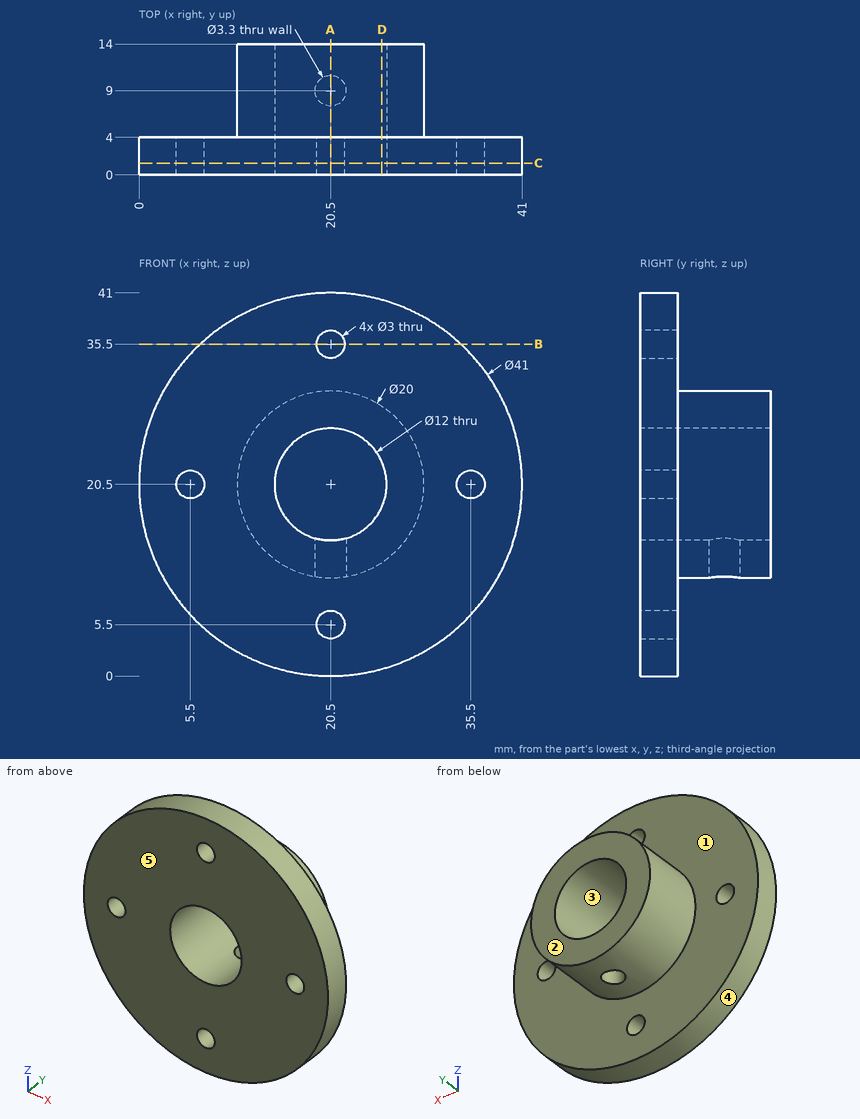
The drawing under review shows one solid part. Ordinate dimensions are in mm from its lowest x, y, z. A direction names the side the tool comes from. Coordinates: 2 decimals unless noted, no trailing zeros. Order: outer loops, then holes, each group sorted by start corner. A loop starts at its lowest first (then second) coordinate and runs counter-clockwise, first axis right, second up. Notation, with made-up numbers: M 56,-6.75 L 106,-6.75 A35 ccw 106,25.25 Z; hole C -30,57 d5. An arc over 180 degrees is marked long. Use a Markdown table: item, result.
(1) Add section B-B (z = 35.5). Give the boundary of the cut face in (x, y), then the cut area to 3 significant figures.
Worked answers:
| item | result |
|---|---|
| outline | M 6.53,0 L 19,0 L 19,4 L 6.53,4 Z; M 22,0 L 34.47,0 L 34.47,4 L 22,4 Z |
| area | 99.8 mm2 |
(2) Wall thickness on probe 1 along X at (y, z) = (3.15, 20.5); probe 2 along Z at (x, y) = (20.5, 7); probe 3 along Y at (x, z) = (20.5, 11.85): over which ranges is each line inside the solid? List them lowest first.
Worked answers:
| item | result |
|---|---|
| probe 1 | x = 0 to 4, 7 to 14.5, 26.5 to 34, 37 to 41 |
| probe 2 | z = 10.5 to 14.5, 26.5 to 30.5 |
| probe 3 | y = 0 to 7.35, 10.65 to 14 |
(3) For the marked faces 1 and 2, list the 3-axis set-ups (+Z, -Z, +X, -X, +Y, -Y) from which the entire face can be reached by the end or side of a thin tool; tool diameter is ignored.
Worked answers:
| item | result |
|---|---|
| face 1 | +Y |
| face 2 | +Z, -Z, +X, -X, +Y |
(4) Draft analysis for pull direction X (two halves, no side actions). For the marked faces 3, 4 and 5, state which applies: released by +X, released by -X, zero draft, split by the parting line, or undercut.
Worked answers:
| item | result |
|---|---|
| face 3 | undercut |
| face 4 | split by the parting line |
| face 5 | zero draft |
(5) Add section C-C (y = 1.25). Give the boundary of the cut face in (x, z).
Worked answers:
| item | result |
|---|---|
| outline | C 20.5,20.5 d41; hole C 5.5,20.5 d3; hole C 20.5,20.5 d12; hole C 20.5,5.5 d3; hole C 20.5,35.5 d3; hole C 35.5,20.5 d3 |
(6) For P1, Ø1, axis at y = 11, z = 11.5, coming from the -X side; P2, Ø1, axis at y = 5.5, z = 19, coming from the -X side; P3, Ø4, axis at x = 20.5, y = 9, coming from the +Z side, all flat-tipped, find the tip position at first contact; note any pin that passes through.
Worked answers:
| item | result |
|---|---|
| P1 | stops at x = 15.23 |
| P2 | stops at x = 10.55 |
| P3 | stops at z = 30.5 |
(7) Add section D-D (x = 26). Give the boundary of the cut face in (y, z).
Worked answers:
| item | result |
|---|---|
| outline | M 0,0.75 L 4,0.75 L 4,12.15 L 14,12.15 L 14,18.1 L 0,18.1 Z; M 0,22.9 L 14,22.9 L 14,28.85 L 4,28.85 L 4,40.25 L 0,40.25 Z |
(8) Add section A-A (x = 20.5). Give the boundary of the cut face in (y, z).
Worked answers:
| item | result |
|---|---|
| outline | M 0,0 L 4,0 L 4,4 L 0,4 Z; M 0,7 L 4,7 L 4,10.5 L 7.35,10.5 L 7.35,14.5 L 0,14.5 Z; M 0,26.5 L 14,26.5 L 14,30.5 L 4,30.5 L 4,34 L 0,34 Z; M 0,37 L 4,37 L 4,41 L 0,41 Z; M 10.65,10.5 L 14,10.5 L 14,14.5 L 10.65,14.5 Z |
